Geometry: final body of the model. Coordinates: model frame, mm. Face numbers are marked on the shaded views. A direction names the side the tool comes from. Round coordinates to 2 decimals unless told otherwise and drop trailing zeros. Loops run counter-clockwise (first coordinate to the right, second up) from the corner with the lowest first, then second, coordinate; pieces in that order, holes last. Notation, with made-up numbers: (-20, 57.5) - (-9, 57.5) arc R20 ccw to (-9, 75.5) - close; hole circle Ø8 at (52.5, 62.5). An arc over 180 degrees is marked (long way). Return JSON: item names as keys, results as strings. Group by question number.
1. Draft query along Z for the marked faces 3, 4 and 5. Return one class per face: +Z half, -Z half, draft (parallel to the pull), parting line (faces both ways), or undercut.
2. Section B-B on z = 0. Return loops of the section in (x, y), and give its area (3 significant figures).
3. Section C-C on x = 0. Return loops of the section in (y, z).
4. First-contact query: pin 1 Ø8 at (y, z) = (16.5, -25.5) entering from +X; pin 2 Ø5 at (x, y) = (-12, 5.5) entering from -Z; pin 3 Ø12 at (x, z) = (-18, 18) entering from +Y. Flat tips, straight axial feed; report the tip coordinate or a pass-through.
5. Material intervals for probe 1 along Y at (x, z) = (5, -21); probe 2 along Z at (x, y) = (-11, 20.5); probe 3 along Z at (x, y) = (-26.5, 4.25), sorted ascending.
6. Section A-A on y = 17.5. Return loops of the section in (x, z) (3 decimals).
7. Set-up query: the marked faces 1 and 2. Return all of +Z, -Z, +X, -X, +Y, -Y with unobstructed straight access to the full face (end or side cutting, diameter ignored); none if empty.
from build123d import *

# Parameters (mm, degrees)
BOSS_EXTRUDE1_DEPTH = 25
BOSS_EXTRUDE2_DEPTH = 25
SKETCH6_R           = 32
CUT_EXTRUDE2_DEPTH  = 24.6
BOSS_EXTRUDE5_DEPTH = 24.6
CIRPATTERN1_COUNT   = 6


with BuildPart() as part:
    # Sketch1 → Boss-Extrude1 (new body)
    with BuildSketch(Plane(origin=(0, 0, 0), x_dir=(1, 0, 0), z_dir=(0, 1, 0))):
        with BuildLine():
            ThreePointArc((1.418185365, -33.998799682), (1.610940688, -34.258772233), (1.922534331, -34.346235045))
            ThreePointArc((1.922534331, -34.346235045), (34.399487229, -0.187825316), (2.297477624, 34.323193275))
            ThreePointArc((2.297477624, 34.323193275), (1.735753357, 34.194354817), (1.33841429, 33.776916))
            ThreePointArc((1.33841429, 33.776916), (0, 32.954150957), (-1.33841429, 33.776916))
            ThreePointArc((-1.33841429, 33.776916), (-1.735753357, 34.194354817), (-2.297477624, 34.323193275))
            ThreePointArc((-2.297477624, 34.323193275), (-34.399545597, -0.176812713), (-1.944525024, -34.344997051))
            ThreePointArc((-1.944525024, -34.344997051), (-1.632875445, -34.257733763), (-1.439953708, -33.997884682))
            ThreePointArc((-1.439953708, -33.997884682), (-0.010549885, -32.954149268), (1.418185365, -33.998799682))
        make_face()
        with BuildLine():
            Line((-2.417, 3.18717916), (0, 3.18717916))
            Line((0, 3.18717916), (2.417, 3.18717916))
            ThreePointArc((2.417, 3.18717916), (0, -4), (-2.417, 3.18717916))
        make_face(mode=Mode.SUBTRACT)
    extrude(amount=BOSS_EXTRUDE1_DEPTH)

    # Sketch5 → Boss-Extrude2 (add)
    with BuildSketch(Plane.XZ):
        with BuildLine():
            Line((-2.732678298, -4.18717916), (0, -4.18717916))
            Line((0, -4.18717916), (2.732678298, -4.18717916))
            ThreePointArc((2.732678298, -4.18717916), (0, 5), (-2.732678298, -4.18717916))
        make_face()
    extrude(amount=-BOSS_EXTRUDE2_DEPTH)

    # Sketch6 → Cut-Extrude2 (cut)
    with BuildSketch(Plane(origin=(0, 25, 0), x_dir=(1, 0, 0), z_dir=(0, 1, 0))):
        Circle(SKETCH6_R)
    extrude(amount=-CUT_EXTRUDE2_DEPTH, mode=Mode.SUBTRACT)

    # Sketch8 → Boss-Extrude5 (add)
    with BuildSketch(Plane(origin=(0, 0.4, 0), x_dir=(1, 0, 0), z_dir=(0, 1, 0))):
        with BuildLine():
            ThreePointArc((3, 31.859064644), (0, 30.3), (-3, 31.859064644))
            ThreePointArc((-3, 31.859064644), (0, 32), (3, 31.859064644))
        make_face()
    boss_extrude5 = extrude(amount=BOSS_EXTRUDE5_DEPTH)

    # CirPattern1: Boss-Extrude5 ×6 about axis
    cirpattern1_axis = Axis((0, 0, 0), (0, 1, 0))
    for i in range(1, CIRPATTERN1_COUNT):
        add(boss_extrude5.rotate(cirpattern1_axis, i * 360 / CIRPATTERN1_COUNT))


solid = part.part
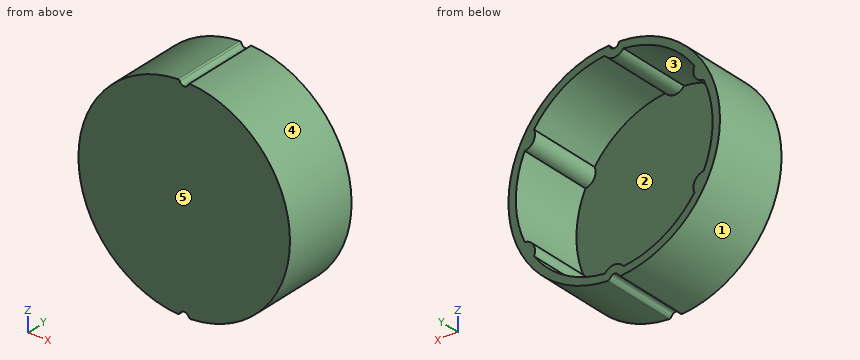
Taken from the geometry:
{
 "1": {"face 3": "undercut", "face 4": "parting line", "face 5": "draft"},
 "2": {"outline": "(-34.4, 0) - (34.4, 0) - (34.4, 25) - (32, 25) - (32, 0.4) - (-32, 0.4) - (-32, 25) - (-34.4, 25) - close", "area": "146 mm2"},
 "3": {"outline": "(0, -32.95) - (25, -32.95) - (25, -30.3) - (0.4, -30.3) - (0.4, 30.3) - (25, 30.3) - (25, 32.95) - (0, 32.95) - close"},
 "4": {"pin 1": "x = 26.85", "pin 2": "z = -33.06", "pin 3": "y = 0.4"},
 "5": {"probe 1": "0 to 0.4", "probe 2": "-32.59 to -30.05, 30.05 to 32.59", "probe 3": "-21.93 to -14.76, 14.76 to 21.93"},
 "6": {"outline": "(-2.297, -34.323) arc R1 ccw to (-1.338, -33.777) arc R1.5 cw to (1.338, -33.777) arc R1 ccw to (2.297, -34.323) arc R34.4 ccw to (1.923, 34.346) arc R0.5 ccw to (1.418, 33.999) arc R1.5 cw to (-1.44, 33.998) arc R0.5 ccw to (-1.945, 34.345) arc R34.4 ccw to start; hole (-29.091, -13.331) arc R3.666 cw to (-26.091, -18.528) arc R32 ccw to (-3, -31.859) arc R3.666 cw to (3, -31.859) arc R32 ccw to (26.091, -18.528) arc R3.666 cw to (29.091, -13.331) arc R32 ccw to (29.091, 13.331) arc R3.666 cw to (26.091, 18.528) arc R32 ccw to (3, 31.859) arc R3.666 cw to (-3, 31.859) arc R32 ccw to (-26.091, 18.528) arc R3.666 cw to (-29.091, 13.331) arc R32 ccw to start"},
 "7": {"face 1": "-X, +Y, -Y", "face 2": "+Y"}
}
